Geometry: final body of the model. Coordinates: model frame, mm. A direction names the side the tool comes from. Give positions to 0.01 mm unless a question says otherwise; leave off trailing zeros. Loops run counter-clockwise (first coordinate to the right, second up) from the corner with the lowest first, then second, coordinate; pieces in that order, holes last. Notation, with made-up numbers: (15, 52) - (31, 52) arc R24 cw to (31, 76) - close; hole circle Ø3 at (49, 32.5). An arc over 180 degrees is marked (long way). Use one line per item in the form item = value.
```python
from build123d import *

# Parameters (mm, degrees)
SKETCH011_W     = 50
SKETCH011_H     = 80
PAD005_DEPTH    = 6
SKETCH012_R     = 1.7
POCKET005_DEPTH = 6
SKETCH013_W     = 7
SKETCH013_H     = 6
POCKET006_DEPTH = 5
SKETCH014_W     = 27
SKETCH014_H     = 27
POCKET007_DEPTH = 5
SKETCH015_W     = 25
SKETCH015_H     = 18.5
POCKET008_DEPTH = 1
POCKET009_DEPTH = 5
POCKET010_DEPTH = 1
SKETCH019_W     = 18
SKETCH019_H     = 5
POCKET011_DEPTH = 3
SKETCH020_W     = 4
SKETCH020_H     = 51
POCKET012_DEPTH = 3
SKETCH021_W     = 5
SKETCH021_H     = 40
POCKET013_DEPTH = 3
SKETCH023_R     = 2.65
POCKET014_DEPTH = 3.2


with BuildPart() as part:
    # Sketch011 → Pad005 (new body)
    with BuildSketch(Plane.XY):
        Rectangle(SKETCH011_W, SKETCH011_H)
    extrude(amount=PAD005_DEPTH)

    # Sketch012 (on Face6 of Pad005) → Pocket005 (cut)
    with BuildSketch(Plane.XY.offset(6)):
        with Locations((-21, 36)):
            Circle(SKETCH012_R)
        with Locations((21, 36)):
            Circle(SKETCH012_R)
        with Locations((-21, -36)):
            Circle(SKETCH012_R)
        with Locations((21, -36)):
            Circle(SKETCH012_R)
    extrude(amount=-POCKET005_DEPTH, mode=Mode.SUBTRACT)

    # Sketch013 (on Face4 of Pocket005) → Pocket006 (cut)
    with BuildSketch(Plane(origin=(0, 0, 0), x_dir=(1, 0, 0), z_dir=(0, 0, -1))):
        with Locations((0, 33.3)):
            Rectangle(SKETCH013_W, SKETCH013_H)
        with Locations((0, 3.3)):
            Rectangle(SKETCH013_W, SKETCH013_H)
        with Locations((0, 18.3)):
            Rectangle(SKETCH013_W, SKETCH013_H)
        with Locations((20, 18.3)):
            Rectangle(SKETCH013_W, SKETCH013_H)
        with Locations((-20, 18.3)):
            Rectangle(SKETCH013_W, SKETCH013_H)
    extrude(amount=-POCKET006_DEPTH, mode=Mode.SUBTRACT)

    # Sketch014 (on Face4 of Pocket006) → Pocket007 (cut)
    with BuildSketch(Plane(origin=(0, 0, 0), x_dir=(1, 0, 0), z_dir=(0, 0, -1))):
        with Locations((0, -24.6)):
            Rectangle(SKETCH014_W, SKETCH014_H)
    extrude(amount=-POCKET007_DEPTH, mode=Mode.SUBTRACT)

    # Sketch015 (on Face40 of Pocket007) → Pocket008 (cut)
    with BuildSketch(Plane(origin=(0, 0, 5), x_dir=(1, 0, 0), z_dir=(0, 0, -1))):
        with Locations((0, -24.85)):
            Rectangle(SKETCH015_W, SKETCH015_H)
    extrude(amount=-POCKET008_DEPTH, mode=Mode.SUBTRACT)

    # Sketch017 (on Face4 of Pocket008) → Pocket009 (cut)
    with BuildSketch(Plane(origin=(0, 0, 0), x_dir=(1, 0, 0), z_dir=(0, 0, -1))):
        Polygon((4.5, 37.5), (-4.5, 37.5), (-4.5, 22.3), (-24, 22.3), (-24, 14.3), (-4.5, 14.3), (-4.5, -0.9), (4.5, -0.9), (4.5, 14.3), (24, 14.3), (24, 22.3), (4.5, 22.3), align=None)
    extrude(amount=-POCKET009_DEPTH, mode=Mode.SUBTRACT)

    # Sketch018 (on Face32 of Pocket009) → Pocket010 (cut)
    with BuildSketch(Plane(origin=(0, 0, 5), x_dir=(1, 0, 0), z_dir=(0, 0, -1))):
        with BuildLine():
            ThreePointArc((0.145291, 29.552816), (1.162743, 36.865183), (-2.326569, 30.358984))
            Line((-2.326569, 30.358984), (-3.72186, 26.080764))
            Line((-3.436646, 25.987745), (-3.72186, 26.080764))
            Line((-1.974516, 30.470904), (-3.436646, 25.987745))
            ThreePointArc((-0.073085, 29.850774), (1.069723, 36.579968), (-1.974516, 30.470904))
            Line((-0.073085, 29.850774), (-1.535215, 25.367615))
            Line((-1.25, 25.274596), (-1.535215, 25.367615))
            Line((0.145291, 29.552816), (-1.25, 25.274596))
        make_face()
        with BuildLine():
            ThreePointArc((-16.482544, 19.6), (-23.75, 18.3), (-16.482544, 17))
            Line((-16.482544, 17), (-11.982544, 17))
            Line((-11.982544, 17), (-11.982544, 17.3))
            Line((-16.698107, 17.3), (-11.982544, 17.3))
            ThreePointArc((-16.698107, 19.3), (-23.45, 18.3), (-16.698107, 17.3))
            Line((-16.698107, 19.3), (-11.982544, 19.3))
            Line((-11.982544, 19.3), (-11.982544, 19.6))
            Line((-16.482544, 19.6), (-11.982544, 19.6))
        make_face()
        with BuildLine():
            ThreePointArc((16.482544, 17), (23.75, 18.3), (16.482544, 19.6))
            Line((16.482544, 19.6), (11.982544, 19.6))
            Line((11.982544, 19.3), (11.982544, 19.6))
            Line((16.698107, 19.3), (11.982544, 19.3))
            ThreePointArc((16.698107, 17.3), (23.45, 18.3), (16.698107, 19.3))
            Line((16.698107, 17.3), (11.982544, 17.3))
            Line((11.982544, 17), (11.982544, 17.3))
            Line((16.482544, 17), (11.982544, 17))
        make_face()
        with BuildLine():
            ThreePointArc((-1.3, 6.817456), (0, -0.45), (1.3, 6.817456))
            Line((1.3, 6.817456), (1.3, 11.317456))
            Line((1.3, 11.317456), (1, 11.317456))
            Line((1, 6.601893), (1, 11.317456))
            ThreePointArc((-1, 6.601893), (0, -0.15), (1, 6.601893))
            Line((-1, 6.601893), (-1, 11.317456))
            Line((-1, 11.317456), (-1.3, 11.317456))
            Line((-1.3, 6.817456), (-1.3, 11.317456))
        make_face()
        with BuildLine():
            ThreePointArc((-0.145291, 22.047184), (-1.162743, 14.734817), (2.326569, 21.241016))
            Line((2.326569, 21.241016), (3.72186, 25.519236))
            Line((3.72186, 25.519236), (3.436646, 25.612255))
            Line((1.974516, 21.129096), (3.436646, 25.612255))
            ThreePointArc((0.073085, 21.749226), (-1.069723, 15.020032), (1.974516, 21.129096))
            Line((0.073085, 21.749226), (1.535215, 26.232385))
            Line((1.535215, 26.232385), (1.25, 26.325404))
            Line((-0.145291, 22.047184), (1.25, 26.325404))
        make_face()
    extrude(amount=-POCKET010_DEPTH, mode=Mode.SUBTRACT)

    # Sketch019 (on Face4 of Pocket010) → Pocket011 (cut)
    with BuildSketch(Plane(origin=(0, 0, 0), x_dir=(1, 0, 0), z_dir=(0, 0, -1))):
        with Locations((0, -4.5)):
            Rectangle(SKETCH019_W, SKETCH019_H)
    extrude(amount=-POCKET011_DEPTH, mode=Mode.SUBTRACT)

    # Sketch020 (on Face4 of Pocket011) → Pocket012 (cut)
    with BuildSketch(Plane(origin=(0, 0, 0), x_dir=(1, 0, 0), z_dir=(0, 0, -1))):
        with Locations((13, 13.7)):
            Rectangle(SKETCH020_W, SKETCH020_H)
    pocket012 = extrude(amount=-POCKET012_DEPTH, mode=Mode.SUBTRACT)

    # Mirrored003: Pocket012 across Sketch020 V_Axis
    add(pocket012.mirror(Plane(origin=(0, 0, 0), x_dir=(0, 0, -1), z_dir=(1, 0, 0))), mode=Mode.SUBTRACT)

    # Sketch021 (on Face4 of Mirrored003) → Pocket013 (cut)
    with BuildSketch(Plane(origin=(0, 0, 0), x_dir=(1, 0, 0), z_dir=(0, 0, -1))):
        with Locations((22.5, -10)):
            Rectangle(SKETCH021_W, SKETCH021_H)
    pocket013 = extrude(amount=-POCKET013_DEPTH, mode=Mode.SUBTRACT)

    # Mirrored004: Pocket013 across Sketch021 V_Axis
    add(pocket013.mirror(Plane(origin=(0, 0, 0), x_dir=(0, 0, -1), z_dir=(1, 0, 0))), mode=Mode.SUBTRACT)

    # Sketch023 (on Face7 of Mirrored004) → Pocket014 (cut)
    with BuildSketch(Plane.XY.offset(6)):
        with Locations((21, 36)):
            Circle(SKETCH023_R)
        with Locations((-21, 36)):
            Circle(SKETCH023_R)
        with Locations((-21, -36)):
            Circle(SKETCH023_R)
        with Locations((21, -36)):
            Circle(SKETCH023_R)
    extrude(amount=-POCKET014_DEPTH, mode=Mode.SUBTRACT)


solid = part.part
```
(1) Cut plane B-B (y = -3.3). Return the cut outline in (x, z), plus the area to 3 significant figures.
Solution:
outline = (-25, 3) - (-20, 3) - (-20, 0) - (-15, 0) - (-15, 3) - (-11, 3) - (-11, 0) - (-4.5, 0) - (-4.5, 5) - (-3.75, 5) - (-3.75, 6) - (-25, 6) - close; (-3.45, 5) - (3.45, 5) - (3.45, 6) - (-3.45, 6) - close; (3.75, 5) - (4.5, 5) - (4.5, 0) - (11, 0) - (11, 3) - (15, 3) - (15, 0) - (20, 0) - (20, 3) - (25, 3) - (25, 6) - (3.75, 6) - close
area = 200 mm2
(2) Cut plane A-A (x = 7). Return the cut outline in (y, z), plus the area to 4 significant figures.
Solution:
outline = (-40, 0) - (-22.3, 0) - (-22.3, 5) - (-14.3, 5) - (-14.3, 0) - (2, 0) - (2, 3) - (7, 3) - (7, 0) - (11.1, 0) - (11.1, 5) - (15.6, 5) - (15.6, 6) - (-40, 6) - close; (34.1, 5) - (38.1, 5) - (38.1, 0) - (40, 0) - (40, 6) - (34.1, 6) - close
area = 271.5 mm2
(3) Material intervals for L1, parallel to Y at x = 21, z = 2.2; L2, parallel to Y at x = 3.5, z = 2.5; L3, parallel to Y at x = 6.5, z = 1.2, sorted ascending. Write a range as from..to.
Solution:
L1 = -40..-37.7, -34.3..-22.3, -14.3..-10, 30..34.3, 37.7..40
L2 = -40..-37.5, 0.9..2, 7..11.1, 38.1..40
L3 = -40..-22.3, -14.3..2, 7..11.1, 38.1..40
(4) Access query for faces 1 (the face through (-22, 10, 3)), 2 (the face through (0.794, -23.959, 5.493)), 3 (the face through (21, -38, 2.8)), 4 (the face through (0, 38.1, 2)). Directions: +Z, -Z, +X, -X, +Y, -Y. A direction counts if a zero-diameter tool reaches every point of the face in a straight line with its end or side. Return the directions, or none.
Solution:
face_1 = -Z, -X
face_2 = +Z, -Z
face_3 = +Z
face_4 = -Z
(5) Cut plane D-D (y = -13). Return the cut outline in (x, z), plus the area to 3 significant figures.
Solution:
outline = (-25, 0) - (-15, 0) - (-15, 3) - (-11, 3) - (-11, 0) - (-4.5, 0) - (-4.5, 5) - (4.5, 5) - (4.5, 0) - (11, 0) - (11, 3) - (15, 3) - (15, 0) - (25, 0) - (25, 6) - (-25, 6) - close
area = 231 mm2
(6) Pin query (flat end, axial travel): P1, Ø1.6, axis at x = -22, y = 37, coming from the +Z side; P2, Ø6, axis at x = 20, y = -18.3, coming from the -Z side; P3, Ø1.5, axis at x = -13.5, y = -4, coming from the -Z side. Return the tip coordinate at first contact, or that it passes through.
Solution:
P1 = 2.8
P2 = 5
P3 = 3
(7) Cut plane C-C (z = 3.8). Return the cut outline in (x, y), plus the area to 3 significant figures.
Solution:
outline = (-25, -40) - (25, -40) - (25, 40) - (-25, 40) - close; hole (-24, -22.3) - (-4.5, -22.3) - (-4.5, -37.5) - (4.5, -37.5) - (4.5, -22.3) - (24, -22.3) - (24, -14.3) - (4.5, -14.3) - (4.5, 0.9) - (-4.5, 0.9) - (-4.5, -14.3) - (-24, -14.3) - close; hole circle Ø5.3 at (-21, -36); hole circle Ø5.3 at (-21, 36); hole (-13.5, 11.1) - (13.5, 11.1) - (13.5, 38.1) - (-13.5, 38.1) - close; hole circle Ø5.3 at (21, -36); hole circle Ø5.3 at (21, 36)
area = 2,530 mm2
